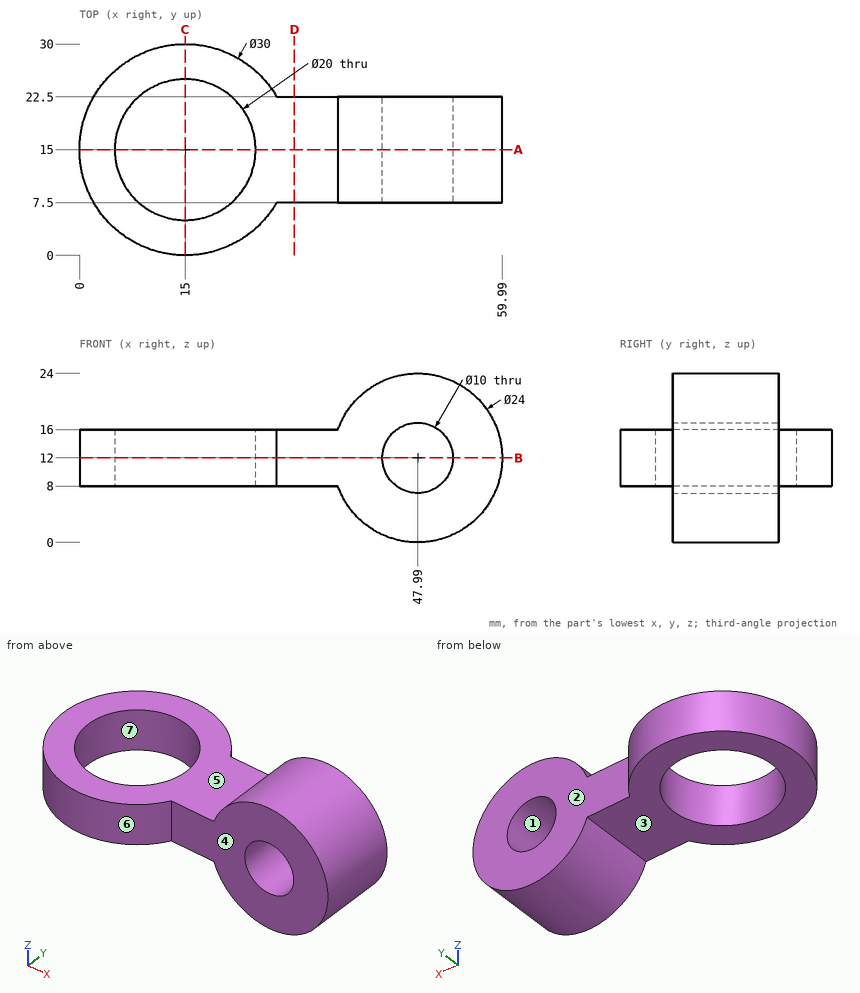
Source: three-view drawing plus pictorial views. Frame: mm from the lowest corner of the part. A direction names the side the tool comes from. Give positions to 0.01 mm unless a question says otherwise; leave off trailing zeros. Loops run counter-clockwise (first coordinate to the right, second up) from the corner with the lowest first, then second, coordinate; pieces in that order, holes last.
1) Mould query, pull axis Y, two halves, no side actions, for the marked faces 5, 6 and 7. Classes: released by +Y, released by -Y, zero draft, split by the parting line, or undercut.
A:
face 5: zero draft
face 6: split by the parting line
face 7: undercut
2) Section query A-A on y = 15. Return the cut outline in (x, z).
A:
outline: (0, 8) - (5, 8) - (5, 16) - (0, 16) - close; (25, 8) - (36.68, 8) arc R12 ccw (long way) to (36.68, 16) - (25, 16) - close; hole circle Ø10 at (47.99, 12)
3) Section query D-D on x = 30.5. Return the cut outline in (y, z).
A:
outline: (7.5, 8) - (22.5, 8) - (22.5, 16) - (7.5, 16) - close
4) Contact query for flat-ended pins moving along their axis: pin 1 (1.5 mm diameter, centred on x = 38, z = 6.5, fed in from +Y); pin 2 (8 mm diameter, centred on x = 18.5, y = 26, fed in from +Z); pin 3 (5 mm diameter, centred on x = 26, y = 18, fed in from -Z). Output: stop coordinate, or through.
A:
pin 1: stops at y = 22.5
pin 2: stops at z = 16
pin 3: stops at z = 8
5) Line query: L1, parallel to X at y = 11, z = 14.25 (1 decimal); L2, parallel to Z at x = 50.5, y = 13.5 (1 decimal); L3, parallel to Z at x = 19, y = 3.5. Output: solid intervals per line, ascending.
A:
L1: x = 0.5 to 5.8, 24.2 to 43.5, 52.5 to 59.8
L2: z = 0.3 to 7.7, 16.3 to 23.7
L3: z = 8 to 16
6) Section query C-C on x = 15. Return the cut outline in (y, z).
A:
outline: (0, 8) - (5, 8) - (5, 16) - (0, 16) - close; (25, 8) - (30, 8) - (30, 16) - (25, 16) - close
7) Section query B-B on z = 12. Return the cut outline in (x, y).
A:
outline: (27.99, 7.5) - (42.99, 7.5) - (42.99, 22.5) - (27.99, 22.5) arc R15 ccw (long way) to start; (52.99, 7.5) - (59.99, 7.5) - (59.99, 22.5) - (52.99, 22.5) - close; hole circle Ø20 at (15, 15)
8) Reachability of the marked faces 1, 2, 3 and 4 from +Z, -Z, +X, -X, +Y, -Y: full face, straight path, thin tool, end or side. Return the list, or none.
A:
face 1: +Y, -Y
face 2: +Z, -Z, +X, +Y
face 3: -Z, -X, +Y, -Y
face 4: +Z, -Z, +X, -Y
